The listing builds one solid part. Answer for the finished solid, in the listing's coordinates (mm). A direction names the side the tool comes from. Give positions to 0.01 mm unless a question says otherwise; leave off trailing zeros. Loops run counter-clockwise (first coordinate to the right, second up) from the corner with the lowest first, then second, coordinate; pieces in that order, holes last.
Item 1: Section A-A, the plane y = -9 is taken. Give the vertices of the cut face in (x, z), and give its area (3 significant figures).
Item 2: Each of these flat-tipped pins is pushed along its axis until it touches: pin 1 Ø3 at (x, y) = (-16, -10) entering from +Z; pin 2 Ø6 at (x, y) = (-1.5, -16) entering from -Z; pin 3 Ø1.5 at (y, z) = (34.5, 0.5) entering from +X; pin 4 Ø1.9 at (x, z) = (0, 1) entering from +Y. Where does it stop, or does it pass through?
Item 3: Consider line 1 along Y through (x, z) = (0, 0.55); line 2 along X through (y, z) = (15.5, 0.25); line 3 along X through (y, z) = (-15, 1.3). Determine where each line is inside the solid, lowest interval first.
Item 4: Section D-D, the plane z = 1.6 is taken. Give the number of separate pieces and of enclosed holes in the cut face, and give its area (3 significant figures).
Item 5: Section B-B, the plane x = 0 is taken. Give the vertices of the cut face in (y, z).
Item 6: Section C-C, the plane y = 36 is taken. Give the vertices of the cut face in (x, z).
Item 7: A tool of negligible diameter and unlimited length cuts with its end or side. For faces 1 (the face through (12.155, -33.768, 1.775)), 2 (the face through (3, -17.8, 1.2)), 3 (the face through (-7.75, 37, 2)), from which of +Z, -Z, +X, -X, +Y, -Y can it reach the whole face along a straight path? Write none if from no direction.
Item 8: The mould has two halves that part along Y. Classify faces 4 (the face through (20, 0, 2)), 5 (the face through (-6.85, 20.86, 1.77)), 6 (the face through (3.8, -47.6, 1.8)), 7 (the face through (-11.46, -33.37, 2.99)): pulls with the +Y half, pulls with the -Y half, needs draft (parallel to the pull), parting line crosses it, or undercut.
from build123d import *

# Parameters (mm, degrees)
F0_R     = 1.7
F0_R_2   = 3.6
F0_R_3   = 6.5
F1_DEPTH = 2.4
F2_DEPTH = 3.6
F3_R     = 1.19999


# Not quite as in the source:
# - a fillet or chamfer is up to 0.001 mm smaller than in the source, because OpenCascade refuses the exact size


with BuildPart() as f1:
    # F0 (on Top) → F1 (new body)
    with BuildSketch(Plane.XY):
        with BuildLine():
            Line((13.3779826676, 50), (14.1634030533, 50.1520355803))
            Line((14.1634030533, 50.1520355803), (13.6953264465, 52.5701334259))
            ThreePointArc((13.6953264465, 52.5701334259), (12.6591358938, 54.3141305363), (10.75, 55))
            ThreePointArc((10.75, 55), (8.6286796564, 54.1213203436), (7.75, 52))
            Line((7.75, 52), (7.75, 50))
            Line((7.75, 50), (8.55, 50))
            Line((8.55, 50), (8.55, 23))
            ThreePointArc((8.55, 23), (7.4370057685, 20.3129942315), (4.75, 19.2))
            Line((4.75, 19.2), (0, 19.2))
            Line((0, 19.2), (-4.75, 19.2))
            ThreePointArc((-4.75, 19.2), (-7.4370057685, 20.3129942315), (-8.55, 23))
            Line((-8.55, 23), (-8.55, 50))
            Line((-8.55, 50), (-7.75, 50))
            Line((-7.75, 50), (-7.75, 52))
            ThreePointArc((-7.75, 52), (-8.6286796564, 54.1213203436), (-10.75, 55))
            ThreePointArc((-10.75, 55), (-12.6591358938, 54.3141305363), (-13.6953264465, 52.5701334259))
            Line((-13.6953264465, 52.5701334259), (-14.1634030533, 50.1520355803))
            Line((-14.1634030533, 50.1520355803), (-13.3779826676, 50))
            Line((-13.3779826676, 50), (-19.1599060608, 20.1304096433))
            ThreePointArc((-19.1599060608, 20.1304096433), (-19.1899535764, 19.9223197335), (-19.2, 19.7123117976))
            Line((-19.2, 19.7123117976), (-19.2, 0))
            Line((-19.2, 0), (-19.2, -19.2052668078))
            ThreePointArc((-19.2, -19.2052668078), (-19.1266435215, -19.768638206), (-18.9114660616, -20.294439657))
            Line((-18.9114660616, -20.294439657), (-4.2133641117, -46.0891728492))
            ThreePointArc((-4.2133641117, -46.0891728492), (-3.4072983694, -46.9021277912), (-2.3018980501, -47.2))
            Line((-2.3018980501, -47.2), (-2.3018980501, -48))
            Line((-2.3018980501, -48), (0, -48))
            Line((0, -48), (2.3018980501, -48))
            Line((2.3018980501, -48), (2.3018980501, -47.2))
            ThreePointArc((2.3018980501, -47.2), (3.4072983694, -46.9021277912), (4.2133641117, -46.0891728492))
            Line((4.2133641117, -46.0891728492), (18.9114660616, -20.294439657))
            ThreePointArc((18.9114660616, -20.294439657), (19.1266435215, -19.768638206), (19.2, -19.2052668078))
            Line((19.2, -19.2052668078), (19.2, 0))
            Line((19.2, 0), (19.2, 19.7123117976))
            ThreePointArc((19.2, 19.7123117976), (19.1899535764, 19.9223197335), (19.1599060608, 20.1304096433))
            Line((19.1599060608, 20.1304096433), (13.3779826676, 50))
        make_face()
        with BuildLine():
            ThreePointArc((-8.6554840981, -29.4059057186), (-9.1040076685, -31.0426178518), (-10.7407198016, -30.5940942814))
            Line((-10.7407198016, -30.5940942814), (-12.721034073, -27.1187014422))
            ThreePointArc((-12.721034073, -27.1187014422), (-12.2725105026, -25.4819893091), (-10.6357983695, -25.9305128794))
            Line((-10.6357983695, -25.9305128794), (-8.6554840981, -29.4059057186))
        make_face(mode=Mode.SUBTRACT)
        with Locations((-15.25, -15.25)):
            Circle(F0_R, mode=Mode.SUBTRACT)
        with BuildLine():
            Line((-6.2, -21), (-6.2, -19))
            ThreePointArc((-6.2, -19), (-5, -17.8), (-3.8, -19))
            Line((-3.8, -19), (-3.8, -21))
            ThreePointArc((-3.8, -21), (-5, -22.2), (-6.2, -21))
        make_face(mode=Mode.SUBTRACT)
        with BuildLine():
            Line((-8.4, 0), (-8.4, 3))
            ThreePointArc((-8.4, 3), (-7.2, 4.2), (-6, 3))
            Line((-6, 3), (-6, 0))
            ThreePointArc((-6, 0), (-7.2, -1.2), (-8.4, 0))
        make_face(mode=Mode.SUBTRACT)
        with BuildLine():
            ThreePointArc((-4, -2.4), (-3.7071067812, -1.6928932188), (-3, -1.4))
            Line((-3, -1.4), (1, -1.4))
            ThreePointArc((1, -1.4), (1.7071067812, -1.6928932188), (2, -2.4))
            Line((2, -2.4), (2, -15.4))
            ThreePointArc((2, -15.4), (1.7071067812, -16.1071067812), (1, -16.4))
            Line((1, -16.4), (-3, -16.4))
            ThreePointArc((-3, -16.4), (-3.7071067812, -16.1071067812), (-4, -15.4))
            Line((-4, -15.4), (-4, -2.4))
        make_face(mode=Mode.SUBTRACT)
        with Locations((0, -45)):
            Circle(F0_R, mode=Mode.SUBTRACT)
        with Locations((0, -37)):
            Circle(F0_R_2, mode=Mode.SUBTRACT)
        with BuildLine():
            Line((12.721034073, -27.1187014422), (10.7407198016, -30.5940942814))
            ThreePointArc((10.7407198016, -30.5940942814), (9.1040076685, -31.0426178518), (8.6554840981, -29.4059057186))
            Line((8.6554840981, -29.4059057186), (10.6357983695, -25.9305128794))
            ThreePointArc((10.6357983695, -25.9305128794), (12.2725105026, -25.4819893091), (12.721034073, -27.1187014422))
        make_face(mode=Mode.SUBTRACT)
        with BuildLine():
            Line((1.8, -21), (1.8, -19))
            ThreePointArc((1.8, -19), (3, -17.8), (4.2, -19))
            Line((4.2, -19), (4.2, -21))
            ThreePointArc((4.2, -21), (3, -22.2), (1.8, -21))
        make_face(mode=Mode.SUBTRACT)
        with Locations((12, -9)):
            Circle(F0_R_3, mode=Mode.SUBTRACT)
        with BuildLine():
            Line((18.8, 3), (18.8, 0))
            ThreePointArc((18.8, 0), (17.6, -1.2), (16.4, 0))
            Line((16.4, 0), (16.4, 3))
            ThreePointArc((16.4, 3), (17.6, 4.2), (18.8, 3))
        make_face(mode=Mode.SUBTRACT)
        with Locations((-15.25, 15.25)):
            Circle(F0_R, mode=Mode.SUBTRACT)
        with Locations((-10.75, 52)):
            Circle(F0_R, mode=Mode.SUBTRACT)
        with Locations((15.25, 15.25)):
            Circle(F0_R, mode=Mode.SUBTRACT)
        with Locations((10.75, 52)):
            Circle(F0_R, mode=Mode.SUBTRACT)
    extrude(amount=F1_DEPTH)

    # F0 (on Top) → F2 (join)
    with BuildSketch(Plane.XY):
        with BuildLine():
            Line((20, -19.2052668078), (20, 0))
            Line((20, 0), (20, 19.7123117976))
            ThreePointArc((20, 19.7123117976), (19.9863003315, 19.9986862557), (19.9453264465, 20.2824452236))
            Line((19.9453264465, 20.2824452236), (14.1634030533, 50.1520355803))
            Line((14.1634030533, 50.1520355803), (13.3779826676, 50))
            Line((13.3779826676, 50), (19.1599060608, 20.1304096433))
            ThreePointArc((19.1599060608, 20.1304096433), (19.1899535764, 19.9223197335), (19.2, 19.7123117976))
            Line((19.2, 19.7123117976), (19.2, 0))
            Line((19.2, 0), (19.2, -19.2052668078))
            ThreePointArc((19.2, -19.2052668078), (19.1266435215, -19.768638206), (18.9114660616, -20.294439657))
            Line((18.9114660616, -20.294439657), (4.2133641117, -46.0891728492))
            ThreePointArc((4.2133641117, -46.0891728492), (3.4072983694, -46.9021277912), (2.3018980501, -47.2))
            Line((2.3018980501, -47.2), (2.3018980501, -48))
            ThreePointArc((2.3018980501, -48), (3.8092621219, -47.5938106244), (4.9084426795, -46.4852357035))
            Line((4.9084426795, -46.4852357035), (19.6065446294, -20.6905025113))
            ThreePointArc((19.6065446294, -20.6905025113), (19.8999684385, -19.9735005326), (20, -19.2052668078))
        make_face()
        with BuildLine():
            Line((8.55, 50), (7.75, 50))
            Line((7.75, 50), (7.75, 23))
            ThreePointArc((7.75, 23), (6.8713203436, 20.8786796564), (4.75, 20))
            Line((4.75, 20), (0, 20))
            Line((0, 20), (-4.75, 20))
            ThreePointArc((-4.75, 20), (-6.8713203436, 20.8786796564), (-7.75, 23))
            Line((-7.75, 23), (-7.75, 50))
            Line((-7.75, 50), (-8.55, 50))
            Line((-8.55, 50), (-8.55, 23))
            ThreePointArc((-8.55, 23), (-7.4370057685, 20.3129942315), (-4.75, 19.2))
            Line((-4.75, 19.2), (0, 19.2))
            Line((0, 19.2), (4.75, 19.2))
            ThreePointArc((4.75, 19.2), (7.4370057685, 20.3129942315), (8.55, 23))
            Line((8.55, 23), (8.55, 50))
        make_face()
        with BuildLine():
            ThreePointArc((-4.9084426795, -46.4852357035), (-3.8092621219, -47.5938106244), (-2.3018980501, -48))
            Line((-2.3018980501, -48), (-2.3018980501, -47.2))
            ThreePointArc((-2.3018980501, -47.2), (-3.4072983694, -46.9021277912), (-4.2133641117, -46.0891728492))
            Line((-4.2133641117, -46.0891728492), (-18.9114660616, -20.294439657))
            ThreePointArc((-18.9114660616, -20.294439657), (-19.1266435215, -19.768638206), (-19.2, -19.2052668078))
            Line((-19.2, -19.2052668078), (-19.2, 0))
            Line((-19.2, 0), (-19.2, 19.7123117976))
            ThreePointArc((-19.2, 19.7123117976), (-19.1899535764, 19.9223197335), (-19.1599060608, 20.1304096433))
            Line((-19.1599060608, 20.1304096433), (-13.3779826676, 50))
            Line((-13.3779826676, 50), (-14.1634030533, 50.1520355803))
            Line((-14.1634030533, 50.1520355803), (-19.9453264465, 20.2824452236))
            ThreePointArc((-19.9453264465, 20.2824452236), (-19.9863003315, 19.9986862557), (-20, 19.7123117976))
            Line((-20, 19.7123117976), (-20, 0))
            Line((-20, 0), (-20, -19.2052668078))
            ThreePointArc((-20, -19.2052668078), (-19.8999684385, -19.9735005326), (-19.6065446294, -20.6905025113))
            Line((-19.6065446294, -20.6905025113), (-4.9084426795, -46.4852357035))
        make_face()
    extrude(amount=F2_DEPTH)

    # F3 (radius 1.2 in the source; OpenCascade refuses exactly that, so slightly less here)
    f3_edges = [f1.edges().sort_by_distance(p)[0] for p in [
        (-13.770693, 50.076018, 3.6),
        (-8.15, 50, 3.6),
        (8.15, 50, 3.6),
        (13.770693, 50.076018, 3.6),
        (-2.301898, -47.6, 3.6),
        (2.301898, -47.6, 3.6),
    ]]
    fillet(f3_edges, radius=F3_R)


solid = f1.part
Worked answers:
1. outline: (-20, 0) - (-4, 0) - (-4, 2.4) - (-19.2, 2.4) - (-19.2, 3.6) - (-20, 3.6) - close; (2, 0) - (5.5, 0) - (5.5, 2.4) - (2, 2.4) - close; (18.5, 0) - (20, 0) - (20, 3.6) - (19.2, 3.6) - (19.2, 2.4) - (18.5, 2.4) - close
1. area: 52.3 mm2
2. pin 1: stops at z = 2.4
2. pin 2: stops at z = 0
2. pin 3: stops at x = 17.34
2. pin 4: stops at y = 20
3. line 1: y = -48 to -46.7, -43.3 to -40.6, -33.4 to -16.4, -1.4 to 20
3. line 2: x = -20 to -16.93, -13.57 to 13.57, 16.93 to 20
3. line 3: x = -20 to -16.93, -13.57 to -4, 2 to 9.5, 14.5 to 20
4. separate pieces: 1
4. enclosed holes: 15
4. area: 2,500 mm2
5. outline: (-48, 0) - (-46.7, 0) - (-46.7, 2.4) - (-48, 2.4) - close; (-43.3, 0) - (-40.6, 0) - (-40.6, 2.4) - (-43.3, 2.4) - close; (-33.4, 0) - (-16.4, 0) - (-16.4, 2.4) - (-33.4, 2.4) - close; (-1.4, 0) - (20, 0) - (20, 3.6) - (19.2, 3.6) - (19.2, 2.4) - (-1.4, 2.4) - close
6. outline: (-16.9, 0) - (-7.75, 0) - (-7.75, 3.6) - (-8.55, 3.6) - (-8.55, 2.4) - (-16.09, 2.4) - (-16.09, 3.6) - (-16.9, 3.6) - close; (7.75, 0) - (16.9, 0) - (16.9, 3.6) - (16.09, 3.6) - (16.09, 2.4) - (8.55, 2.4) - (8.55, 3.6) - (7.75, 3.6) - close
7. face 1: +Z, -Z, +X, -Y
7. face 2: +Z, -Z
7. face 3: +Z, -Z, +Y
8. face 4: needs draft
8. face 5: pulls with the +Y half
8. face 6: pulls with the -Y half
8. face 7: undercut
